Answer from the drawing. Dimensions are ordinates in mm from the lowest x, y and z of the part. A direction names the side the tool comes from. Round coordinates to 2 decimals unless told otherwise and drop trailing zeros. Write each loop counter-clockwise with the first axis right and the second up, starting at its lowest first coordinate (ties: lowest second). Pieces come first, ordered by that corner, then holes. Notation, with made-up numbers: (51, 76) - (92, 76) arc R20 ccw to (92, 84) - close; hole circle Ø11 at (83, 77). An arc over 180 degrees is marked (long way). Answer as CSV lines item,"result". Start each with the question number.
1) Consider line 1 along Y through (x, z) = (0.5, 3.5); line 2 along Y through (x, z) = (1, 3); line 3 along X through (y, z) = (39.5, 2.25). Determine where each line is inside the solid, lowest interval first.
2) Find section A-A on x = 4. Determine the outline of the cut face in (y, z), then the cut area to 3 significant figures.
3) Which of the six approach directions +Z, -Z, +X, -X, +Y, -Y give full straight-line access (tool end or side, diameter ignored) to the marked faces 1 and 2?
4) Find section C-C on y = 3.5. Determine the outline of the cut face in (x, z).
5) Each of these flat-tipped pins is pushed along its axis until it touches: pin 1 (1 mm diameter, centred on y = 20, z = 3, fed in from -X); pin 2 (2 mm diameter, centred on x = 1.5, y = 20.5, fed in from +Z). Where does it stop, or does it pass through?
6) Find section B-B on z = 4. Determine the outline of the cut face in (x, y).
7) Find section D-D on z = 7. Determine the outline of the cut face in (x, y).
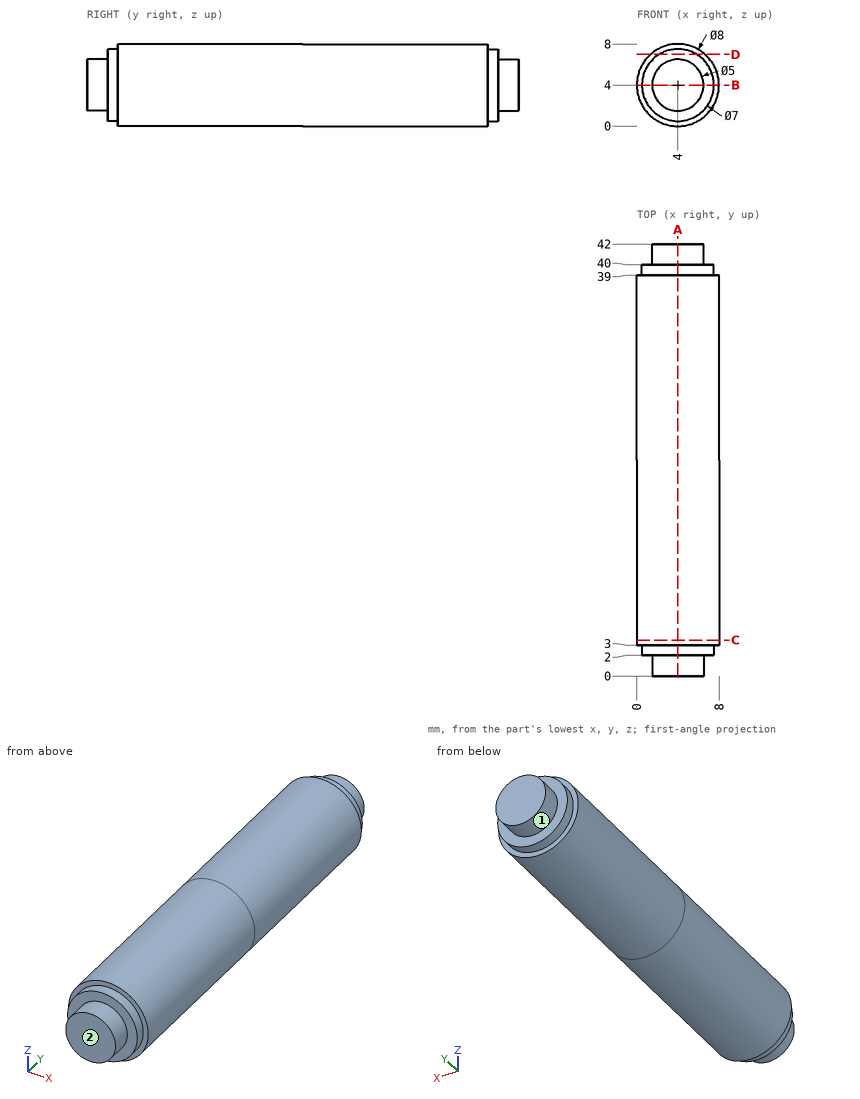
Check values:
1,line 1,"y = 3 to 39"
1,line 2,"y = 2 to 40"
1,line 3,"x = 0.97 to 7.03"
2,outline,"(0, 1.5) - (2, 1.5) - (2, 0.5) - (3, 0.5) - (3, 0) - (39, 0) - (39, 0.5) - (40, 0.5) - (40, 1.5) - (42, 1.5) - (42, 6.5) - (40, 6.5) - (40, 7.5) - (39, 7.5) - (39, 8) - (3, 8) - (3, 7.5) - (2, 7.5) - (2, 6.5) - (0, 6.5) - close"
2,area,"322 mm^2"
3,face 1,"+Y"
3,face 2,"+Z, -Z, +X, -X, -Y"
4,outline,"circle Ø8 at (4, 4)"
5,pin 1,"stops at x = 0.03"
5,pin 2,"stops at z = 7.71"
6,outline,"(0, 3) - (0.5, 3) - (0.5, 2) - (1.5, 2) - (1.5, 0) - (6.5, 0) - (6.5, 2) - (7.5, 2) - (7.5, 3) - (8, 3) - (8, 39) - (7.5, 39) - (7.5, 40) - (6.5, 40) - (6.5, 42) - (1.5, 42) - (1.5, 40) - (0.5, 40) - (0.5, 39) - (0, 39) - close"
7,outline,"(1.35, 3) - (2.2, 3) - (2.2, 2) - (5.8, 2) - (5.8, 3) - (6.65, 3) - (6.65, 39) - (5.8, 39) - (5.8, 40) - (2.2, 40) - (2.2, 39) - (1.35, 39) - close"
